Check sheet for the modelled part. Datum: model origin and axes. Units: mm. Face numbers are marked on the shaded views. A direction names the side the tool comes from. Coordinates: 2 decimals unless noted, no trailing zeros. Write each loop counter-clockwise with the first axis right and the second up, starting at its lowest first coordinate (ties: lowest second). Pieces come first, ordered by that corner, then holes. Notation, with made-up numbers: (43.5, 16) - (60.5, 16) arc R21 ccw to (60.5, 32) - close; hole circle Ø1 at (45.25, 62). An arc over 180 degrees is marked (long way). Write each question's results on one line, items separated by ' | '.
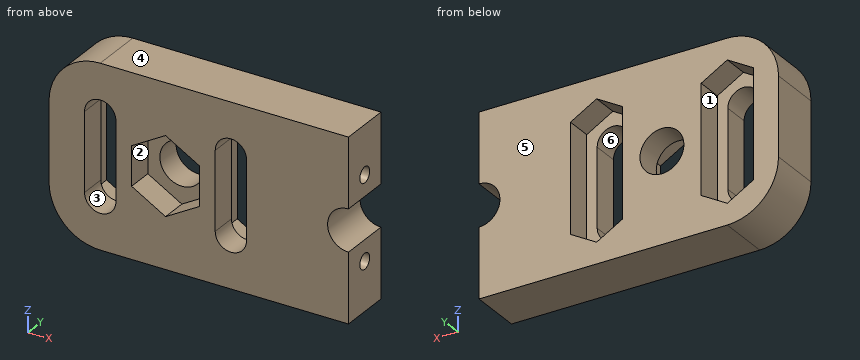
from build123d import *

# Parameters (mm, degrees)
SKETCH_R             = 4.2
PAD_DEPTH            = 10
POCKET_DEPTH         = 5
POCKET001_DEPTH      = 5
SKETCH003_R          = 1.5
POCKET002_DEPTH      = 10
BODY_PLACEMENT_ANGLE = 270


with BuildPart() as part:
    # Sketch → Pad (new body)
    with BuildSketch(Plane.XY):
        with BuildLine():
            ThreePointArc((-22.3, -7.500028), (-19.429637, -14.429656), (-12.5, -17.3))
            Line((-12.5, -17.3), (35, -17.3))
            Line((35, -4), (35, -17.3))
            ThreePointArc((35, 4), (31, 0), (35, -4))
            Line((35, 4), (35, 17.3))
            Line((-12.5, 17.3), (35, 17.3))
            ThreePointArc((-12.5, 17.3), (-19.429639, 14.429654), (-22.3, 7.500021))
            Line((-22.3, -7.500028), (-22.3, 7.500021))
        make_face()
        Circle(SKETCH_R, mode=Mode.SUBTRACT)
        with BuildLine():
            ThreePointArc((-15.5, -7.5), (-12.5, -10.5), (-9.5, -7.5))
            Line((-9.5, -7.5), (-9.5, 7.5))
            ThreePointArc((-9.5, 7.5), (-12.5, 10.5), (-15.5, 7.5))
            Line((-15.5, -7.5), (-15.5, 7.5))
        make_face(mode=Mode.SUBTRACT)
        with BuildLine():
            ThreePointArc((9.5, -7.5), (12.5, -10.5), (15.5, -7.5))
            Line((15.5, -7.5), (15.5, 7.5))
            ThreePointArc((15.5, 7.5), (12.5, 10.5), (9.5, 7.5))
            Line((9.5, -7.5), (9.5, 7.5))
        make_face(mode=Mode.SUBTRACT)
    extrude(amount=PAD_DEPTH)

    # Sketch001 (on Face19 of Pad) → Pocket (cut)
    with BuildSketch(Plane.XY.offset(10)):
        Polygon((-12.5, 13.273503), (-17.5, 10.386751), (-17.5, 4.613249), (-17.5, -4.613249), (-17.5, -10.386751), (-12.5, -13.273503), (-7.5, -10.386751), (-7.5, -4.613249), (-7.5, 4.613249), (-7.5, 10.386751), align=None)
        Polygon((7.5, -4.613249), (7.5, -10.386751), (12.5, -13.273503), (17.5, -10.386751), (17.5, -4.613249), (17.5, 4.613249), (17.5, 10.386751), (12.5, 13.273503), (7.5, 10.386751), (7.5, 4.613249), align=None)
    extrude(amount=-POCKET_DEPTH, mode=Mode.SUBTRACT)

    # Sketch002 → Pocket001 (cut)
    with BuildSketch(Plane.XY):
        Polygon((-6.5, 3.752777), (-6.5, -3.752777), (0, -7.505553), (6.5, -3.752777), (6.5, 3.752777), (0, 7.505553), align=None)
    extrude(amount=POCKET001_DEPTH, mode=Mode.SUBTRACT)

    # Sketch003 (on Face10 of Pocket001) → Pocket002 (cut)
    with BuildSketch(Plane.YZ.offset(35)):
        with Locations((-8, 5)):
            Circle(SKETCH003_R)
        with Locations((8, 5)):
            Circle(SKETCH003_R)
    extrude(amount=-POCKET002_DEPTH, mode=Mode.SUBTRACT)


with BuildPart() as part_1:
    # Body placement: moved
    add(part.part.moved(Location((0, 0, 15))).rotate(Axis((0, 0, 15), (1, 0, 0)), BODY_PLACEMENT_ANGLE))


solid = part_1.part
1. Draft check along Z on the marked faces 4, 5 and 6. Enter one of: pulls with the +Z half, pulls with the -Z half, needs draft (parallel to the pull), parting line crosses it, or undercut.
Values follow:
face 4: pulls with the +Z half | face 5: needs draft | face 6: undercut
2. Go/stop test with flat-tipped pins: pin 1 (2.5 mm diameter, centred on y = 3, z = 15, fed in from +X); pin 2 (0.9 mm diameter, centred on y = 5, z = 23.5, fed in from +X); pin 3 (5 mm diameter, centred on x = -14, z = 14.5, fed in from +Y). Record where each tip stops, or that it passes through.
Values follow:
pin 1: stops at x = 31.2 | pin 2: stops at x = 25 | pin 3: stops at y = 5
3. Sectioned sample at D-D (z = 29.5). Record the cut outline in (x, y).
Values follow:
outline: (-19.36, 0) - (35, 0) - (35, 10) - (-19.36, 10) - close
4. Sectioned sample at B-B (z = 15). Record the cut outline in (x, y), then the cut area to 3 significant figures.
Values follow:
outline: (-22.3, 0) - (-15.5, 0) - (-15.5, 5) - (-17.5, 5) - (-17.5, 10) - (-22.3, 10) - close; (-9.5, 0) - (-6.5, 0) - (-6.5, 5) - (-4.2, 5) - (-4.2, 10) - (-7.5, 10) - (-7.5, 5) - (-9.5, 5) - close; (4.2, 5) - (6.5, 5) - (6.5, 0) - (9.5, 0) - (9.5, 5) - (7.5, 5) - (7.5, 10) - (4.2, 10) - close; (15.5, 0) - (31, 0) - (31, 10) - (17.5, 10) - (17.5, 5) - (15.5, 5) - close | area: 266 mm^2
5. Material ranges on L1, parallel to X at y = 8.25, z = 10; L2, parallel to X at y = 8.5, z = 15; L3, parallel to Y at x = 32, z = 7, recorded low to high. Write a range as [from, to].
Values follow:
L1: x = [-22.3, -17.5], [-7.5, 7.5], [17.5, 35] | L2: x = [-22.3, -17.5], [-7.5, -4.2], [4.2, 7.5], [17.5, 31] | L3: y = [0, 3.5], [6.5, 10]
6. Access from +Z, -Z, +X, -X, +Y, -Y to the whole of each face (thin tool, end or side, straight path). Record for the marked faces 1, 2 and 3.
Values follow:
face 1: +Y | face 2: -Y | face 3: +Y, -Y
7. Sectioned sample at C-C (y = 1.5). Record the cut outline in (x, z).
Values follow:
outline: (-22.3, 7.5) arc R9.8 ccw to (-12.5, -2.3) - (35, -2.3) - (35, 11) arc R4 cw to (35, 19) - (35, 32.3) - (-12.5, 32.3) arc R9.8 ccw to (-22.3, 22.5) - close; hole (-15.5, 7.5) arc R3 ccw to (-9.5, 7.5) - (-9.5, 22.5) arc R3 ccw to (-15.5, 22.5) - close; hole (-6.5, 11.25) - (0, 7.49) - (6.5, 11.25) - (6.5, 18.75) - (0, 22.51) - (-6.5, 18.75) - close; hole (9.5, 7.5) arc R3 ccw to (15.5, 7.5) - (15.5, 22.5) arc R3 ccw to (9.5, 22.5) - close
8. Sectioned sample at A-A (y = 9). Record the cut outline in (x, z), then the cut area to 3 significant figures.
Values follow:
outline: (-22.3, 7.5) arc R9.8 ccw to (-12.5, -2.3) - (35, -2.3) - (35, 11) arc R4 cw to (35, 19) - (35, 32.3) - (-12.5, 32.3) arc R9.8 ccw to (-22.3, 22.5) - close; hole (-17.5, 4.61) - (-12.5, 1.73) - (-7.5, 4.61) - (-7.5, 25.39) - (-12.5, 28.27) - (-17.5, 25.39) - close; hole circle Ø8.4 at (0, 15); hole (7.5, 4.61) - (12.5, 1.73) - (17.5, 4.61) - (17.5, 25.39) - (12.5, 28.27) - (7.5, 25.39) - close | area: 1,390 mm^2
